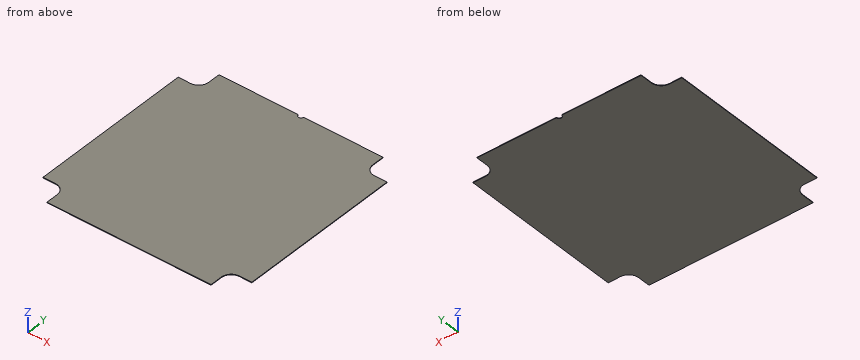
from build123d import *

# Parameters (mm, degrees)
FE_00082_OUTLINE_R = 3.3782
FE_00082_DEPTH     = 6.35
SKETCH1_W          = 5.588
SKETCH1_H          = 266.7
CUT_EXTRUDE1_DEPTH = 299.247271572
CUT_EXTRUDE2_DEPTH = 189.586918009


# Read off the part's stored shape, not the designer's step: FE-00082
with BuildPart() as part:
    # FE-00082 outline → FE-00082 (new body)
    with BuildSketch(Plane.XY):
        with BuildLine():
            Line((127, 133.35), (4.62461393, 133.35))
            ThreePointArc((4.62461393, 133.35), (3.702137995, 133.054473064), (3.123115901, 132.277922078))
            ThreePointArc((3.123115901, 132.277922078), (0, 130.048), (-3.123115901, 132.277922078))
            ThreePointArc((-3.123115901, 132.277922078), (-3.702137995, 133.054473064), (-4.62461393, 133.35))
            Line((-4.62461393, 133.35), (-127, 133.35))
            ThreePointArc((-127, 133.35), (-131.490128061, 131.490128061), (-133.35, 127))
            Line((-133.35, 127), (-133.35, -127))
            ThreePointArc((-133.35, -127), (-131.490128061, -131.490128061), (-127, -133.35))
            Line((-127, -133.35), (127, -133.35))
            ThreePointArc((127, -133.35), (131.490128061, -131.490128061), (133.35, -127))
            Line((133.35, -127), (133.35, 127))
            ThreePointArc((133.35, 127), (131.490128061, 131.490128061), (127, 133.35))
        make_face()
        with Locations((-117.475, -117.475)):
            Circle(FE_00082_OUTLINE_R, mode=Mode.SUBTRACT)
        with Locations((117.475, -117.475)):
            Circle(FE_00082_OUTLINE_R, mode=Mode.SUBTRACT)
        with Locations((-117.475, 117.475)):
            Circle(FE_00082_OUTLINE_R, mode=Mode.SUBTRACT)
        with Locations((117.475, 117.475)):
            Circle(FE_00082_OUTLINE_R, mode=Mode.SUBTRACT)
    extrude(amount=FE_00082_DEPTH)

    # Sketch1 → Cut-Extrude1 (cut, through all)
    with BuildSketch(Plane(origin=(133.35, 0, 0), x_dir=(0, 0, -1), z_dir=(1, 0, 0))):
        with Locations((-2.794, 0)):
            Rectangle(SKETCH1_W, SKETCH1_H)
    extrude(amount=-CUT_EXTRUDE1_DEPTH, mode=Mode.SUBTRACT)

    # Sketch2 → Cut-Extrude2 (cut, through all)
    with BuildSketch(Plane.XY.offset(6.35)):
        with BuildLine():
            Line((-133.35, 104.775), (-117.475, 104.775))
            ThreePointArc((-117.475, 104.775), (-108.494743879, 108.494743879), (-104.775, 117.475))
            Line((-104.775, 117.475), (-104.775, 133.35))
            Line((-104.775, 133.35), (-127, 133.35))
            ThreePointArc((-127, 133.35), (-131.490128061, 131.490128061), (-133.35, 127))
            Line((-133.35, 127), (-133.35, 104.775))
        make_face()
        with BuildLine():
            Line((-104.775, -133.35), (-127, -133.35))
            ThreePointArc((-127, -133.35), (-131.490128061, -131.490128061), (-133.35, -127))
            Line((-133.35, -127), (-133.35, -104.775))
            Line((-133.35, -104.775), (-117.475, -104.775))
            ThreePointArc((-117.475, -104.775), (-108.494743879, -108.494743879), (-104.775, -117.475))
            Line((-104.775, -117.475), (-104.775, -133.35))
        make_face()
        with BuildLine():
            Line((133.35, -104.775), (117.475, -104.775))
            ThreePointArc((117.475, -104.775), (108.494743879, -108.494743879), (104.775, -117.475))
            Line((104.775, -117.475), (104.775, -133.35))
            Line((104.775, -133.35), (127, -133.35))
            ThreePointArc((127, -133.35), (131.490128061, -131.490128061), (133.35, -127))
            Line((133.35, -127), (133.35, -104.775))
        make_face()
        with BuildLine():
            Line((104.775, 133.35), (127, 133.35))
            ThreePointArc((127, 133.35), (131.490128061, 131.490128061), (133.35, 127))
            Line((133.35, 127), (133.35, 104.775))
            Line((133.35, 104.775), (117.475, 104.775))
            ThreePointArc((117.475, 104.775), (108.494743879, 108.494743879), (104.775, 117.475))
            Line((104.775, 117.475), (104.775, 133.35))
        make_face()
    extrude(amount=-CUT_EXTRUDE2_DEPTH, mode=Mode.SUBTRACT)


solid = part.part
Read the model definition and answer for the solid it produces. Units are mm, in the model's axes. Round coordinates to 2 decimals unless told otherwise and drop trailing zeros. Loops run counter-clockwise (first coordinate to the right, second up) from the corner with the lowest first, then second, coordinate; pieces in that order, holes last. Notation, with made-up numbers: (53, -14) - (102, -14) arc R22 cw to (102, -1) - close; hole circle Ø11 at (52, 86.5). An arc over 180 degrees is marked (long way). One line per question, with ' | ' between items. Start each with the question number.
Q1. Section B-B on x = 114 is taken. Give the vertices of the cut face in (y, z).
Q2. Section C-C on y = -113 is taken. Give the vertices of the cut face in (x, z), plus the area to 3 significant figures.
Q3. Find the intervals of material crossed by L1, parallel to Y at x = 120, z = 6.3 (3 decimals); L2, parallel to X at y = 112, z = 5.85, in increasing order.
Established:
1) outline: (-105.26, 5.59) - (105.26, 5.59) - (105.26, 6.35) - (-105.26, 6.35) - close
2) outline: (-105.59, 5.59) - (105.59, 5.59) - (105.59, 6.35) - (-105.59, 6.35) - close | area: 161 mm²
3) L1: -104.775 to 104.775 | L2: -106.02 to 106.02
